The drawing under review shows one solid part. Ordinate dimensions are in mm from its lowest x, y, z. A direction names the side the tool comes from. Coordinates: 2 decimals unless noted, no trailing zeros. Loops run counter-clockwise (first coordinate to the right, second up) from the corner with the lowest first, then second, coordinate; pieces in that order, holes last. Notation, with made-up numbers: M -20.75,-37 L 15.25,-37 A19 ccw 15.25,-15 Z; hole C 20,69 d2. An arc over 180 degrees is marked long. Return JSON: item names as keys, results as strings.
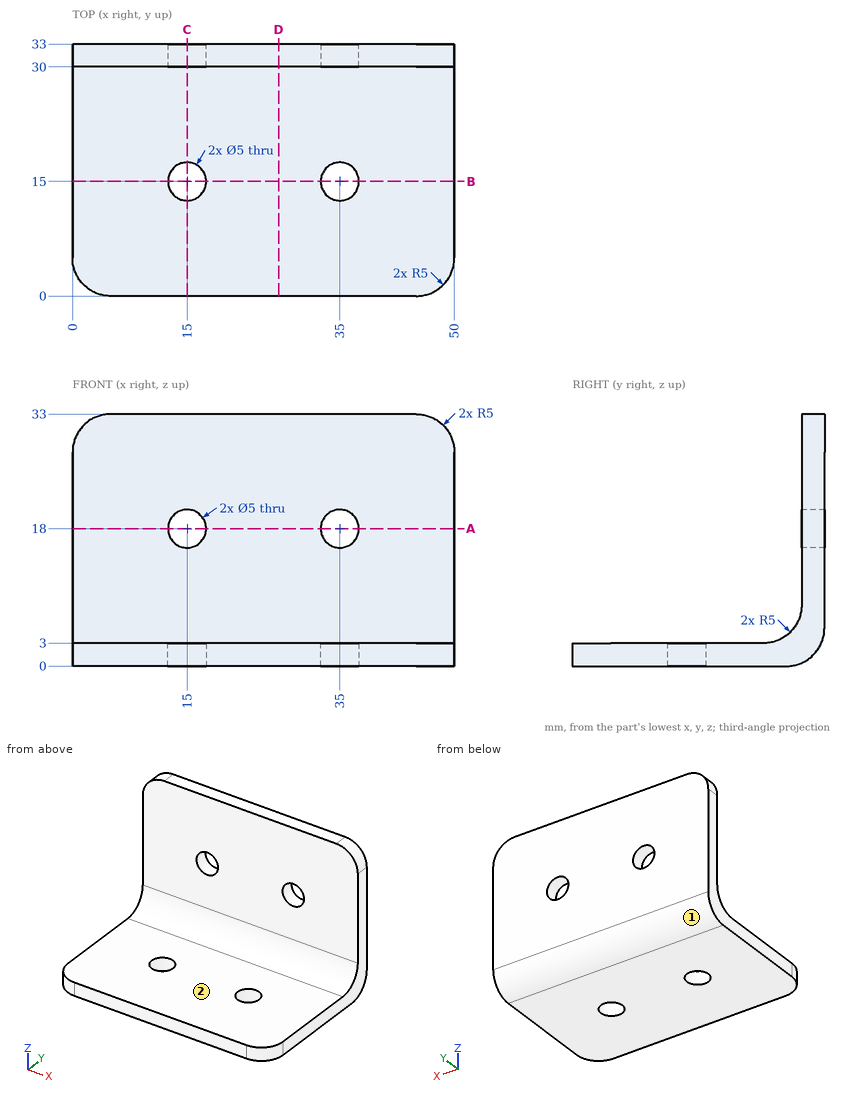
1. Add section A-A on z = 18. Give the boundary of the cut face in (x, y), plus the area to 3 significant figures.
Check values:
{"outline": "M 0,30 L 12.5,30 L 12.5,33 L 0,33 Z; M 17.5,30 L 32.5,30 L 32.5,33 L 17.5,33 Z; M 37.5,30 L 50,30 L 50,33 L 37.5,33 Z", "area": "120 mm²"}
2. Add section C-C on x = 15. Give the boundary of the cut face in (y, z), plus the area to 3 significant figures.
Check values:
{"outline": "M 0,0 L 12.5,0 L 12.5,3 L 0,3 Z; M 17.5,0 L 28,0 A5 ccw 33,5 L 33,15.5 L 30,15.5 L 30,8 A5 cw 25,3 L 17.5,3 Z; M 30,20.5 L 33,20.5 L 33,33 L 30,33 Z", "area": "159 mm²"}
3. To check wall thickness, follow line 1 (X direction, y = 31.6, z = 18); line 2 (Y direction, x = 19, z = 27); line 3 (Z direction, x = 16, y = 20). State the ranges of each line that lie inside material, in increasing order.
Check values:
{"line 1": "0 to 12.5, 17.5 to 32.5, 37.5 to 50", "line 2": "30 to 33", "line 3": "0 to 3"}
4. Machinability: for the marked faces 1 and 2, which of the approach directions +Z, -Z, +X, -X, +Y, -Y give a long, thin tool a straight path to every point of the face, cutting with its end or side? Answer none if there is none.
Check values:
{"face 1": "-Z, +X, -X, +Y", "face 2": "+Z, +X, -X, -Y"}
5. Add section D-D on x = 27. Give the boundary of the cut face in (y, z), plus the area to 3 significant figures.
Check values:
{"outline": "M 0,0 L 28,0 A5 ccw 33,5 L 33,33 L 30,33 L 30,8 A5 cw 25,3 L 0,3 Z", "area": "189 mm²"}
6. Add section B-B on y = 15. Give the boundary of the cut face in (x, z).
Check values:
{"outline": "M 0,0 L 12.5,0 L 12.5,3 L 0,3 Z; M 17.5,0 L 32.5,0 L 32.5,3 L 17.5,3 Z; M 37.5,0 L 50,0 L 50,3 L 37.5,3 Z"}
7. Insertion check: pin 1 Ø4 at (x, y) = (35, 15) entering from -Z; pin 2 Ø12.5 at (x, z) = (32, 19.5) entering from -Y; pin 3 Ø8 at (x, y) = (15, 15) entering from +Z; pin 4 Ø12 at (x, z) = (6, 11.5) entering from -Y. Each pin has a flat end and moves straight along its axis. Give the tip position at first contact, or say it passes through.
Check values:
{"pin 1": "through", "pin 2": "y = 30", "pin 3": "z = 3", "pin 4": "y = 29.33"}
